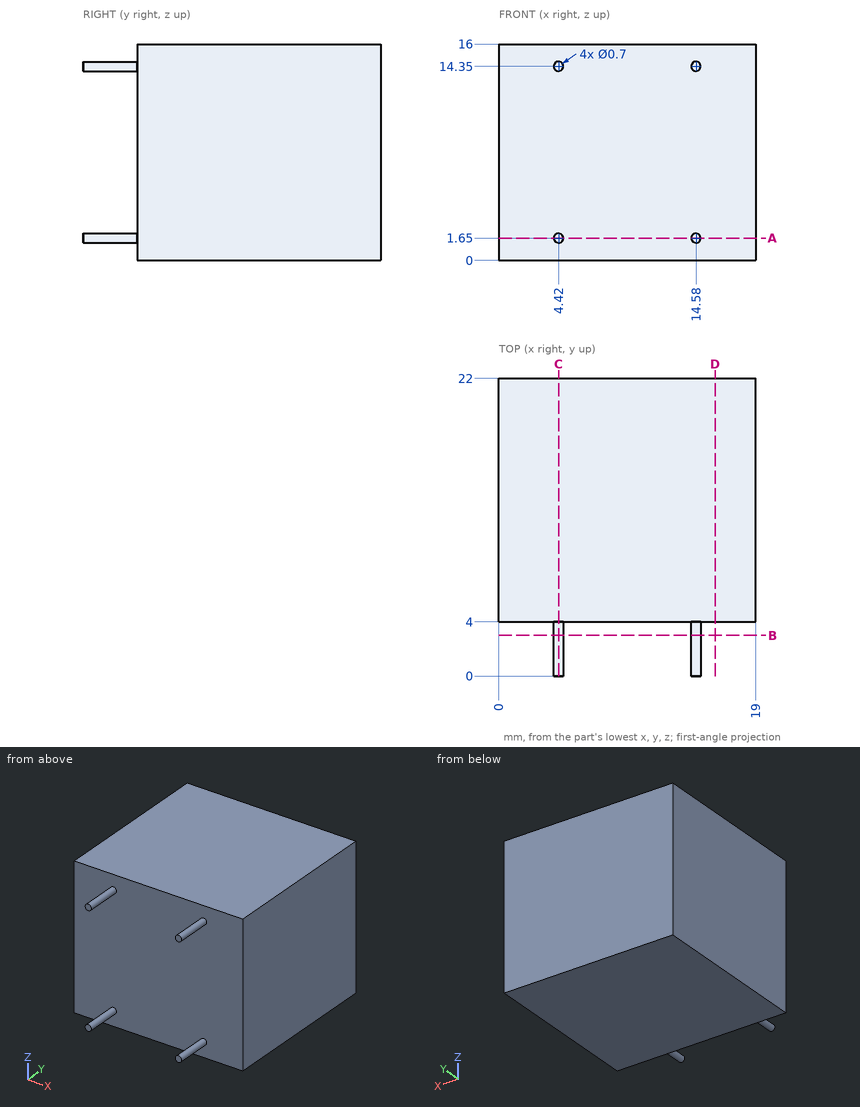
Study the drawing (mm; zero at the part's minimum x, y, z) and answer. Give positions to 0.01 mm unless a question says otherwise; leave off trailing zeros. Write each loop counter-clockwise with the first axis right and the second up, starting at its lowest first coordinate (ties: lowest second). Pieces come first, ordered by that corner, then holes.
(1) The part is cut by section A-A on z = 1.65. Write down the section's boundary in (x, y).
Final values:
outline: (0, 4) - (4.07, 4) - (4.07, 0) - (4.77, 0) - (4.77, 4) - (14.23, 4) - (14.23, 0) - (14.93, 0) - (14.93, 4) - (19, 4) - (19, 22) - (0, 22) - close
(2) The part is cut by section B-B on y = 3. Write down the section's boundary in (x, z).
Final values:
outline: circle Ø0.7 at (4.42, 1.65); circle Ø0.7 at (4.42, 14.35); circle Ø0.7 at (14.58, 1.65); circle Ø0.7 at (14.58, 14.35)
(3) Flat-ended cylindrical pins translate along their axes: pin 1 Ø2 at (y, z) = (2.5, 7) entering from +X; pin 2 Ø1 at (x, z) = (12.5, 10.5) entering from -Y. Find the tip coordinate at first contact, or state that the pin passes through.
Final values:
pin 1: passes through
pin 2: stops at y = 4
(4) The part is cut by section D-D on x = 16. Write down the section's boundary in (y, z).
Final values:
outline: (4, 0) - (22, 0) - (22, 16) - (4, 16) - close
(5) The part is cut by section C-C on x = 4.42. Write down the section's boundary in (y, z).
Final values:
outline: (0, 1.3) - (4, 1.3) - (4, 0) - (22, 0) - (22, 16) - (4, 16) - (4, 14.7) - (0, 14.7) - (0, 14) - (4, 14) - (4, 2) - (0, 2) - close
(6) A straight line is drawn through the part: line 1 (Y direction, x = 6, z = 11.5). Find the intervals that lie inside material, in ascending order.
Final values:
line 1: y = 4 to 22
